```python
from build123d import *

# Parameters (mm, degrees)
SKETCH1_R                       = 15.08125
BOSS_EXTRUDE1_DEPTH             = 6.35
SKETCH4_R                       = 3.3655
CUT_EXTRUDE1_DEPTH              = 885.657788357
CIRPATTERN1_COUNT               = 6
CIRPATTERN1_ANGLE               = 60.5
CIRPATTERN1_THE_OTHER_WAY_COUNT = 6
CIRPATTERN1_THE_OTHER_WAY_ANGLE = 60.5
F_1_4_0_25_DIAMETER_SLOT1_DEPTH = 6.35
CUT_EXTRUDE2_DEPTH              = 885.657788357
FILLET2_R                       = 9.525
FILLET3_R                       = 12.7
SKETCH9_W                       = 6.35
SKETCH9_H                       = 346.075
CUT_EXTRUDE3_DEPTH              = 3.175
FILLET4_R                       = 9.525


# Read off the part's stored shape, not the designer's step: 1/4 (0.25) Diameter Slot1
with BuildPart() as part:
    # Sketch1 → Boss-Extrude1 (new body)
    with BuildSketch(Plane(origin=(0, 0, 0), x_dir=(0, 0, -1), z_dir=(1, 0, 0))):
        with BuildLine():
            Line((-558.8, 609.6), (-558.8, 685.8))
            Line((-558.8, 685.8), (558.8, 685.8))
            Line((558.8, 685.8), (558.8, 609.6))
            ThreePointArc((558.8, 609.6), (494.720400534, 431.550891286), (331.874551798, 335.171901195))
            Line((331.874551798, 335.171901195), (173.0375, 304.8))
            Line((173.0375, 304.8), (-173.0375, 304.8))
            Line((-173.0375, 304.8), (-331.874551798, 335.171901195))
            ThreePointArc((-331.874551798, 335.171901195), (-494.720400534, 431.550891286), (-558.8, 609.6))
        make_face()
        with Locations((-508, 647.7)):
            Circle(SKETCH1_R, mode=Mode.SUBTRACT)
        with Locations((508, 647.7)):
            Circle(SKETCH1_R, mode=Mode.SUBTRACT)
    extrude(amount=BOSS_EXTRUDE1_DEPTH)

    # Sketch4 → Cut-Extrude1 (cut, through all)
    with BuildSketch(Plane(origin=(6.35, 0, 0), x_dir=(0, 0, -1), z_dir=(1, 0, 0))):
        with Locations((0, 345.954707227)):
            Circle(SKETCH4_R)
        with Locations((0, 330.079707227)):
            Circle(SKETCH4_R)
    cut_extrude1 = extrude(amount=-CUT_EXTRUDE1_DEPTH, mode=Mode.SUBTRACT)

    # CirPattern1: Cut-Extrude1 ×6 about axis
    cirpattern1_axis = Axis((0, 909.517207227, 0), (1, 0, 0))
    for i in range(1, CIRPATTERN1_COUNT):
        add(cut_extrude1.rotate(cirpattern1_axis, i * CIRPATTERN1_ANGLE / (CIRPATTERN1_COUNT - 1)), mode=Mode.SUBTRACT)

    # CirPattern1 the other way: Cut-Extrude1 ×6 about axis
    cirpattern1_the_other_way_axis = Axis((0, 909.517207227, 0), (-1, 0, 0))
    for i in range(1, CIRPATTERN1_THE_OTHER_WAY_COUNT):
        add(cut_extrude1.rotate(cirpattern1_the_other_way_axis, i * CIRPATTERN1_THE_OTHER_WAY_ANGLE / (CIRPATTERN1_THE_OTHER_WAY_COUNT - 1)), mode=Mode.SUBTRACT)

    # 1/4 (0.25) Diameter Slot1 outline → 1/4 (0.25) Diameter Slot1 (cut)
    with BuildSketch(Plane.YZ):
        with BuildLine():
            Line((539.75, 152.4), (527.05, 152.4))
            ThreePointArc((527.05, 152.4), (523.875, 149.225), (527.05, 146.05))
            Line((527.05, 146.05), (539.75, 146.05))
            ThreePointArc((539.75, 146.05), (542.925, 149.225), (539.75, 152.4))
        make_face()
        with BuildLine():
            ThreePointArc((387.35, 152.4), (384.175, 149.225), (387.35, 146.05))
            Line((387.35, 146.05), (400.05, 146.05))
            ThreePointArc((400.05, 146.05), (403.225, 149.225), (400.05, 152.4))
            Line((400.05, 152.4), (387.35, 152.4))
        make_face()
        with BuildLine():
            Line((539.75, 184.15), (527.05, 184.15))
            ThreePointArc((527.05, 184.15), (523.875, 180.975), (527.05, 177.8))
            Line((527.05, 177.8), (539.75, 177.8))
            ThreePointArc((539.75, 177.8), (542.925, 180.975), (539.75, 184.15))
        make_face()
        with BuildLine():
            ThreePointArc((387.35, 184.15), (384.175, 180.975), (387.35, 177.8))
            Line((387.35, 177.8), (400.05, 177.8))
            ThreePointArc((400.05, 177.8), (403.225, 180.975), (400.05, 184.15))
            Line((400.05, 184.15), (387.35, 184.15))
        make_face()
    f_1_4_0_25_diameter_slot1 = extrude(amount=F_1_4_0_25_DIAMETER_SLOT1_DEPTH, mode=Mode.SUBTRACT)

    # Mirror1: 1/4 (0.25) Diameter Slot1 across plane
    add(f_1_4_0_25_diameter_slot1.mirror(Plane.XY), mode=Mode.SUBTRACT)

    # Sketch7 → Cut-Extrude2 (cut, through all)
    with BuildSketch(Plane(origin=(6.35, 0, 0), x_dir=(0, 0, -1), z_dir=(1, 0, 0))):
        with BuildLine():
            Line((-179.3875, 254), (-179.3875, 355.6))
            ThreePointArc((-179.3875, 355.6), (-176.2125, 358.775), (-173.0375, 355.6))
            Line((-173.0375, 355.6), (-173.0375, 254))
            ThreePointArc((-173.0375, 254), (-176.2125, 250.825), (-179.3875, 254))
        make_face()
    cut_extrude2 = extrude(amount=-CUT_EXTRUDE2_DEPTH, mode=Mode.SUBTRACT)

    # Mirror5: Cut-Extrude2 across plane
    add(cut_extrude2.mirror(Plane.XY), mode=Mode.SUBTRACT)

    # Fillet2
    fillet2_edges = [part.edges().sort_by_distance(p)[0] for p in [
        (3.175, 306.014210226, 179.3875),
        (3.175, 306.014210226, -179.3875),
    ]]
    fillet(fillet2_edges, radius=FILLET2_R)

    # Fillet3
    fillet3_edges = [part.edges().sort_by_distance(p)[0] for p in [
        (3.175, 685.8, 558.8),
        (3.175, 685.8, -558.8),
    ]]
    fillet(fillet3_edges, radius=FILLET3_R)

    # Sketch9 → Cut-Extrude3 (cut)
    with BuildSketch(Plane.XZ.offset(-304.8)):
        with Locations((3.175, 0)):
            Rectangle(SKETCH9_W, SKETCH9_H)
    extrude(amount=-CUT_EXTRUDE3_DEPTH, mode=Mode.SUBTRACT)

    # Fillet4
    fillet4_edges = [part.edges().sort_by_distance(p)[0] for p in [
        (3.175, 307.975, 173.0375),
        (3.175, 307.975, -173.0375),
    ]]
    fillet(fillet4_edges, radius=FILLET4_R)


solid = part.part
```
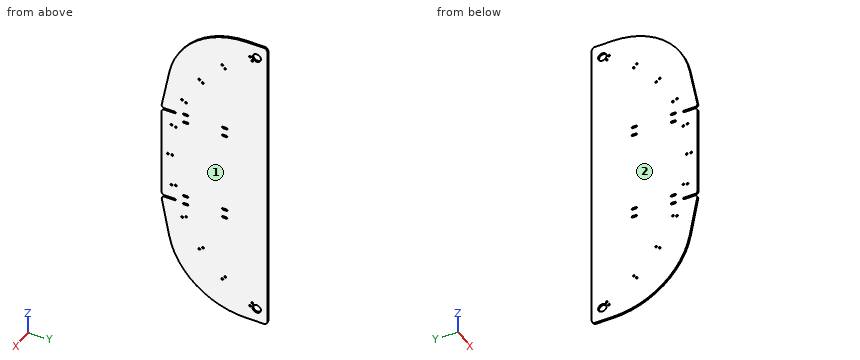
Input: part model. Units: mm. Frame: model coordinates. Face numbers are marked on the shaded views. Round coordinates to 2 decimals unless told otherwise and drop trailing zeros. Write each loop counter-clockwise with the first axis right and the second up, starting at its lowest first coordinate (ties: lowest second). Pieces come first, ordered by that corner, then holes. Notation, with made-up numbers: M 33,-40 L 65,-40 A25 ccw 65,-26 Z; hole C -29.75,11.25 d11. An arc over 180 degrees is marked long. Write each question's results on one line, items separated by ' | '.
Q1. Section query C-C (z = 319.5). Return loops of the section in (x, y).
Results:
outline: M 0,332.81 L 6.35,332.81 L 6.35,685.8 L 0,685.8 Z
Q2. Pin query (flat end, axial travel): P1, Ø5.5, axis at y = 632.01, z = -490.5, coming from the -X side; P2, Ø1.5, axis at x = 1, y = 489, coming from the +Z side; P3, Ø3, axis at x = 2, y = 396, coming from the -Z side. Return the tip coordinate at first contact, or that it passes through.
Results:
P1: passes through | P2: stops at z = 531.79 | P3: stops at z = -461.27
Q3. Section query D-D (z = -407.5). Return loops of the section in (x, y).
Results:
outline: M 0,361.3 L 6.35,361.3 L 6.35,685.8 L 0,685.8 Z
Q4. Section query A-A (y = 647.7). Return loops of the section in (x, z), and give its area (3 significant figures).
Results:
outline: M 0,-558.8 L 6.35,-558.8 L 6.35,-523.08 L 0,-523.08 Z; M 0,-492.92 L 6.35,-492.92 L 6.35,492.92 L 0,492.92 Z; M 0,523.08 L 6.35,523.08 L 6.35,558.8 L 0,558.8 Z | area: 6,710 mm^2
Q5. Section query B-B (x = 1.25). State how many separate pieces and enclosed holes the cut face has, and give its area (3 significant figures).
Results:
separate pieces: 1 | enclosed holes: 32 | area: 371,000 mm^2
Q6. Line query: line 1 along Z through (x, y) = (5.25, 647.7); line 2 along Y through (x, z) = (3, 0) (3 decimals); line 3 along Z through (x, y) = (4, 440). Output: solid intervals per line, ascending.
Results:
line 1: z = -558.8 to -523.08, -492.92 to 492.92, 523.08 to 558.8 | line 2: y = 307.975 to 326.714, 333.445 to 342.589, 349.32 to 685.8 | line 3: z = -501.44 to -345.25, -340.82 to 340.82, 345.25 to 501.44
Q7. Draft query along X for the marked faces 1 and 2. Return one class per face: released by +X, released by -X, zero draft, split by the parting line, or undercut.
Results:
face 1: released by +X | face 2: released by -X
